```python
from build123d import *

# Parameters (mm, degrees)
SKETCH1_W           = 75
SKETCH1_H           = 35
SKETCH1_R           = 7.5
SKETCH1_R_2         = 4
BOSS_EXTRUDE1_DEPTH = 20
SKETCH2_W           = 12
SKETCH2_H           = 23.5
CUT_EXTRUDE1_DEPTH  = 15
SKETCH3_R           = 5
CUT_EXTRUDE2_DEPTH  = 46.961940777


with BuildPart() as part:
    # Sketch1 → Boss-Extrude1 (new body)
    with BuildSketch(Plane(origin=(0, 0, 0), x_dir=(1, 0, 0), z_dir=(0, 1, 0))):
        Rectangle(SKETCH1_W, SKETCH1_H)
        with Locations(Location((24.087416082, 0.196874766, 0), (0, 0, 270))):
            Circle(SKETCH1_R, mode=Mode.SUBTRACT)
        with Locations(Location((-27.5, 0.196874766, 0), (0, 0, 270))):
            Circle(SKETCH1_R_2, mode=Mode.SUBTRACT)
    extrude(amount=BOSS_EXTRUDE1_DEPTH)

    # Sketch2 → Cut-Extrude1 (cut)
    with BuildSketch(Plane(origin=(0, 20, 0), x_dir=(1, 0, 0), z_dir=(0, 1, 0))):
        with Locations((-27.5, 5.75)):
            Rectangle(SKETCH2_W, SKETCH2_H)
    extrude(amount=-CUT_EXTRUDE1_DEPTH, mode=Mode.SUBTRACT)

    # Sketch3 → Cut-Extrude2 (cut, through all)
    with BuildSketch(Plane(origin=(0, 20, 0), x_dir=(1, 0, 0), z_dir=(0, 1, 0))):
        with Locations(Location((0.5, 6.5, 0), (0, 0, 270))):
            Circle(SKETCH3_R)
    extrude(amount=-CUT_EXTRUDE2_DEPTH, mode=Mode.SUBTRACT)


solid = part.part
```
Design review of the part built by this model. Coordinates are the model's own, in mm. A direction names the side the tool comes from. Coordinates: 2 decimals unless noted, no trailing zeros. Loops run counter-clockwise (first coordinate to the right, second up) from the corner with the lowest first, then second, coordinate; pieces in that order, holes last.
Q1. The part is to be moulded in two halves that separate along Z. For faces 3 (the face through (-21.5, 13, -6)), 4 (the face through (2, 10.14, -1.73)), 5 (the face through (-1, 10, 17.5)), say which applies: +Z half, -Z half, draft (parallel to the pull), parting line (faces both ways), or undercut.
Reported:
face 3: draft
face 4: undercut
face 5: +Z half
Q2. We need section C-C on y = 8.75. State the section outline as (x, z) points.
Reported:
outline: (-37.5, -17.5) - (-33.5, -17.5) - (-33.5, 6) - (-21.5, 6) - (-21.5, -17.5) - (37.5, -17.5) - (37.5, 17.5) - (-37.5, 17.5) - close; hole circle Ø10 at (0.5, -6.5); hole circle Ø15 at (24.09, -0.2)
Q3. We need section D-D on z = -13. State the section outline as (x, y) points.
Reported:
outline: (-37.5, 0) - (37.5, 0) - (37.5, 20) - (-21.5, 20) - (-21.5, 5) - (-33.5, 5) - (-33.5, 20) - (-37.5, 20) - close
Q4. Tool access review of faces 1 (the face through (16.766, 9.86, -1.823)), 2 (the face through (-28, 13, 6)): name each direction out of +Z, -Z, +X, -X, +Y, -Y from which nothing blocks a thin tool from reaching the whole face with its end or side.
Reported:
face 1: +Y, -Y
face 2: -Z, +Y
Q5. We need section B-B on z = -9. State the section outline as (x, y) points, and give its area (3 significant figures).
Reported:
outline: (-37.5, 0) - (-3.83, 0) - (-3.83, 20) - (-21.5, 20) - (-21.5, 5) - (-33.5, 5) - (-33.5, 20) - (-37.5, 20) - close; (4.83, 0) - (37.5, 0) - (37.5, 20) - (4.83, 20) - close
area: 1,150 mm2
Q6. We need section A-A on x = 0.5. State the section outline as (y, z) points.
Reported:
outline: (0, -17.5) - (20, -17.5) - (20, -11.5) - (0, -11.5) - close; (0, -1.5) - (20, -1.5) - (20, 17.5) - (0, 17.5) - close
Q7. To check wall thickness, follow line 1 (X direction, y = 2.5, z = 0); line 2 (X direction, y = 5.5, z = 4.5); line 3 (X direction, y = 7.5, z = -6.5). State the ranges of each line that lie inside material, in increasing order.
Reported:
line 1: x = -37.5 to -31.5, -23.5 to 16.59, 31.58 to 37.5
line 2: x = -37.5 to -33.5, -21.5 to 18.24, 29.93 to 37.5
line 3: x = -37.5 to -33.5, -21.5 to -4.5, 5.5 to 20.02, 28.15 to 37.5
Q8. For pin 1 (6 mm diameter, centred on x = -26, z = -6.5, fed in from +Y); pin 2 (5 mm diameter, centred on x = 16.5, z = 5.5, fed in from -Y); pin 3 (3.5 mm diameter, centred on x = -28.5, y = 9.5, fed in from -Z), all flat-tipped, find the tip position at first contact; note any pin that passes through.
Reported:
pin 1: stops at y = 5
pin 2: stops at y = 0
pin 3: stops at z = 6
